from build123d import *

# Parameters (mm, degrees)
SKETCH1_R            = 3.75
BOSS_EXTRUDE1_DEPTH  = 150
LPATTERN1_COUNT      = 2
LPATTERN1_PITCH      = 76.2
LPATTERN1_COUNT_DIR2 = 2
LPATTERN1_PITCH_DIR2 = 25.4
LPATTERN2_COUNT      = 2
LPATTERN2_PITCH      = 14
LPATTERN2_COUNT_DIR2 = 2
LPATTERN2_PITCH_DIR2 = 31.5
LPATTERN3_COUNT      = 2
LPATTERN3_PITCH      = 16
LPATTERN3_COUNT_DIR2 = 2
LPATTERN3_PITCH_DIR2 = 25
SKETCH6_W            = 63.5
SKETCH6_H            = 60
BOSS_EXTRUDE2_DEPTH  = 10
CUT_EXTRUDE1_DEPTH   = 7
SKETCH8_W            = 7.25
SKETCH8_H            = 34
CUT_EXTRUDE2_DEPTH   = 13


with BuildPart() as part:
    # Sketch1 → Boss-Extrude1 (new body)
    with BuildSketch(Plane(origin=(0, 0, 0), x_dir=(1, 0, 0), z_dir=(0, 1, 0))):
        with BuildLine():
            ThreePointArc((-31.75, -6), (-37.75, 0), (-31.75, 6))
            Line((-31.75, 6), (0, 6))
            Line((0, 6), (0, -6))
            Line((0, -6), (-31.75, -6))
        make_face()
        with Locations((-31.75, 0)):
            Circle(SKETCH1_R, mode=Mode.SUBTRACT)
    boss_extrude1 = extrude(amount=BOSS_EXTRUDE1_DEPTH)

    # Mirror1: Boss-Extrude1 across plane
    add(boss_extrude1.mirror(Plane(origin=(0, 150, 0), x_dir=(0, 0, 1), z_dir=(-1, 0, 0))))

    # Sketch2 → Cut-Revolve1 (revolve, cut)
    with BuildSketch(Plane(origin=(12.7, 0, -12.7), x_dir=(0, 0, 1), z_dir=(-1, 0, 0))):
        Polygon((6.2, 65), (15.599823137, 65), (15.599823137, 62.75), (11.59988209, 62.771716936), (8.19988209, 62.321716936), (6.2, 62.3), align=None)
    cut_revolve1 = revolve(axis=Axis((12.7, 65, -6.5), (0, 0, 1)), mode=Mode.SUBTRACT)

    # LPattern1: Cut-Revolve1 2 × 2
    with Locations(*[(-j * LPATTERN1_PITCH_DIR2, i * LPATTERN1_PITCH, 0) for i in range(LPATTERN1_COUNT) for j in range(LPATTERN1_COUNT_DIR2) if (i, j) != (0, 0)]):
        add(cut_revolve1, mode=Mode.SUBTRACT)

    # Sketch3 → Cut-Revolve2 (revolve, cut)
    with BuildSketch(Plane(origin=(15.75, 0, 3.05), x_dir=(0, 0, 1), z_dir=(-1, 0, 0))):
        Polygon((-9.55, 20), (-0.150176863, 20), (-0.150176863, 17.75), (-4.15011791, 17.771716936), (-7.55011791, 17.321716936), (-9.55, 17.3), align=None)
    cut_revolve2 = revolve(axis=Axis((15.75, 20, -6.5), (0, 0, 1)), mode=Mode.SUBTRACT)

    # LPattern2: Cut-Revolve2 2 × 2
    with Locations(*[(-j * LPATTERN2_PITCH_DIR2, i * LPATTERN2_PITCH, 0) for i in range(LPATTERN2_COUNT) for j in range(LPATTERN2_COUNT_DIR2) if (i, j) != (0, 0)]):
        add(cut_revolve2, mode=Mode.SUBTRACT)

    # Sketch4 → Cut-Revolve3 (revolve, cut)
    with BuildSketch(Plane(origin=(12.5, 0, 15.55), x_dir=(0, 0, 1), z_dir=(-1, 0, 0))):
        Polygon((-9.05, 77), (-18.449823137, 77), (-18.449823137, 79.25), (-14.44988209, 79.228283064), (-11.04988209, 79.678283064), (-9.05, 79.7), align=None)
    cut_revolve3 = revolve(axis=Axis((12.5, 77, 6.5), (0, 0, -1)), mode=Mode.SUBTRACT)

    # LPattern3: Cut-Revolve3 2 × 2
    with Locations(*[(-j * LPATTERN3_PITCH_DIR2, i * LPATTERN3_PITCH, 0) for i in range(LPATTERN3_COUNT) for j in range(LPATTERN3_COUNT_DIR2) if (i, j) != (0, 0)]):
        add(cut_revolve3, mode=Mode.SUBTRACT)

    # Sketch6 → Boss-Extrude2 (add)
    with BuildSketch(Plane.XY.offset(6)):
        with Locations((0, 30)):
            Rectangle(SKETCH6_W, SKETCH6_H)
    extrude(amount=BOSS_EXTRUDE2_DEPTH)

    # Sketch7 → Cut-Extrude1 (cut)
    with BuildSketch(Plane.XY.offset(6)):
        Polygon((-2, 3), (-31.75, 3), (-31.75, 57), (-31.75, 60), (-24.75, 60), (-24.75, 57), (-2, 57), align=None)
    cut_extrude1 = extrude(amount=CUT_EXTRUDE1_DEPTH, mode=Mode.SUBTRACT)

    # Mirror2: Cut-Extrude1 across plane
    add(cut_extrude1.mirror(Plane(origin=(0, 0, 0), x_dir=(0, 0, 1), z_dir=(1, 0, 0))), mode=Mode.SUBTRACT)

    # Sketch8 → Cut-Extrude2 (cut, through all)
    with BuildSketch(Plane.XY.offset(6)):
        with Locations((-23.125, 79.5)):
            Rectangle(SKETCH8_W, SKETCH8_H)
    cut_extrude2 = extrude(amount=-CUT_EXTRUDE2_DEPTH, mode=Mode.SUBTRACT)

    # Mirror3: Cut-Extrude2 across plane
    add(cut_extrude2.mirror(Plane(origin=(0, 0, 0), x_dir=(0, 0, 1), z_dir=(1, 0, 0))), mode=Mode.SUBTRACT)


solid = part.part
The model under review builds one solid part; all positions refer to its coordinate system, in mm. A direction names the side the tool comes from. Round coordinates to 2 decimals unless told otherwise and drop trailing zeros. Loops run counter-clockwise (first coordinate to the right, second up) from the corner with the lowest first, then second, coordinate; pieces in that order, holes last. Notation, with made-up numbers: (24, 10.5) -> (51, 10.5) arc R36 cw to (51, 46.5) -> close; hole circle Ø3 at (-25.75, 1.5). An arc over 180 degrees is marked (long way). One line per question, with ' | ' between items. Start each with the question number.
Item 1: Add section B-B, the plane y = 11.5. Write out the cut boundary in (x, z).
Item 2: Draft analysis for pull direction Z (two halves, no side actions). For faces 4 (the face through (-14.635, 94.11, 2.446)), 5 (the face through (-31.75, 22.9, 13.2)), 6 (the face through (-18.133, 18.76, -5.261)), 7 (the face through (14.72, 76.71, -0.87)), state which applies: +Z half, -Z half, draft (parallel to the pull), parting line (faces both ways), or undercut.
Item 3: Add section D-D, the plane y = 131.5. Write out the cut boundary in (x, z).
Item 4: For pin 1 (3 mm diameter, centred on x = 0, z = 9, fed in from +Y); pin 2 (3.5 mm diameter, centred on y = 58, z = 10.5, fed in from +X); pin 3 (10 mm diameter, centred on x = -15, y = 80.5, fed in from +Z), all flat-tipped, find the tip position at first contact; note any pin that passes through.
Item 5: Add section C-C, the plane z = 9.25. Write out the cut boundary in (x, y).
Item 6: Add section A-A, the plane x = 22.5. Write out the cut boundary in (y, z).
Item 7: Wall thickness on line 1 along X through (y, z) = (106, 0); line 2 along Y through (x, z) = (-14, 4.75); line 3 along X through (y, z) = (70, 0): over which ranges is each line inside the solid? List them lowest first. Write a range as [from, to].
Item 8: Machinability: for faces 1 (the face through (-17, 3, 9)), 2 (the face through (-15.632, 36.684, -5.261)), 3 (the face through (-11.69, 95.56, 5.26)), which of the approach directions +Z, -Z, +X, -X, +Y, -Y give a long, thin tool a straight path to every point of the face, cutting with its end or side? Answer none if there is none.
Return value:
1) outline: (-31.75, -6) -> (31.75, -6) arc R6 ccw to (31.75, 6) -> (2, 6) -> (2, 13) -> (31.75, 13) -> (31.75, 16) -> (-31.75, 16) -> (-31.75, 13) -> (-2, 13) -> (-2, 6) -> (-31.75, 6) arc R6 ccw to start; hole circle Ø7.5 at (-31.75, 0); hole circle Ø7.5 at (31.75, 0)
2) face 4: +Z half | face 5: draft | face 6: -Z half | face 7: undercut
3) outline: (-31.75, -6) -> (31.75, -6) arc R6 ccw to (31.75, 6) -> (-31.75, 6) arc R6 ccw to start; hole circle Ø7.5 at (-31.75, 0); hole circle Ø7.5 at (31.75, 0)
4) pin 1: stops at y = 60 | pin 2: stops at x = 24.75 | pin 3: stops at z = 6
5) outline: (-31.75, 0) -> (31.75, 0) -> (31.75, 3) -> (2, 3) -> (2, 57) -> (24.75, 57) -> (24.75, 60) -> (-24.75, 60) -> (-24.75, 57) -> (-2, 57) -> (-2, 3) -> (-31.75, 3) -> close
6) outline: (0, -6) -> (62.5, -6) -> (62.5, 6) -> (60, 6) -> (60, 16) -> (0, 16) -> close; (96.5, -6) -> (150, -6) -> (150, 6) -> (96.5, 6) -> close; hole (3, 6) -> (57, 6) -> (57, 13) -> (3, 13) -> close
7) line 1: x = [-37.75, -35.5], [-28, 28], [35.5, 37.75] | line 2: y = [0, 74.78], [79.22, 90.78], [95.22, 150] | line 3: x = [-37.75, -35.5], [-28, -26.75], [-19.5, 19.5], [26.75, 28], [35.5, 37.75]
8) face 1: -X | face 2: -Z | face 3: +Z
